Job drawing, mm, ordinate dimensions from the low corner. One solid piece. A direction names the side the tool comes from. Coordinates: 2 decimals unless noted, no trailing zeros. Write each loop counter-clockwise with the first axis right and the second up, starting at its lowest first coordinate (ties: lowest second). Pieces come first, ordered by that corner, then holes. Notation, with made-up numbers: (58.5, 74) - (77.5, 74) arc R17 ccw to (77.5, 93) - close; hole circle Ø3 at (52.25, -10). An arc over 180 degrees is marked (long way). Use one line per item in the form item = value. Start each with the question number.
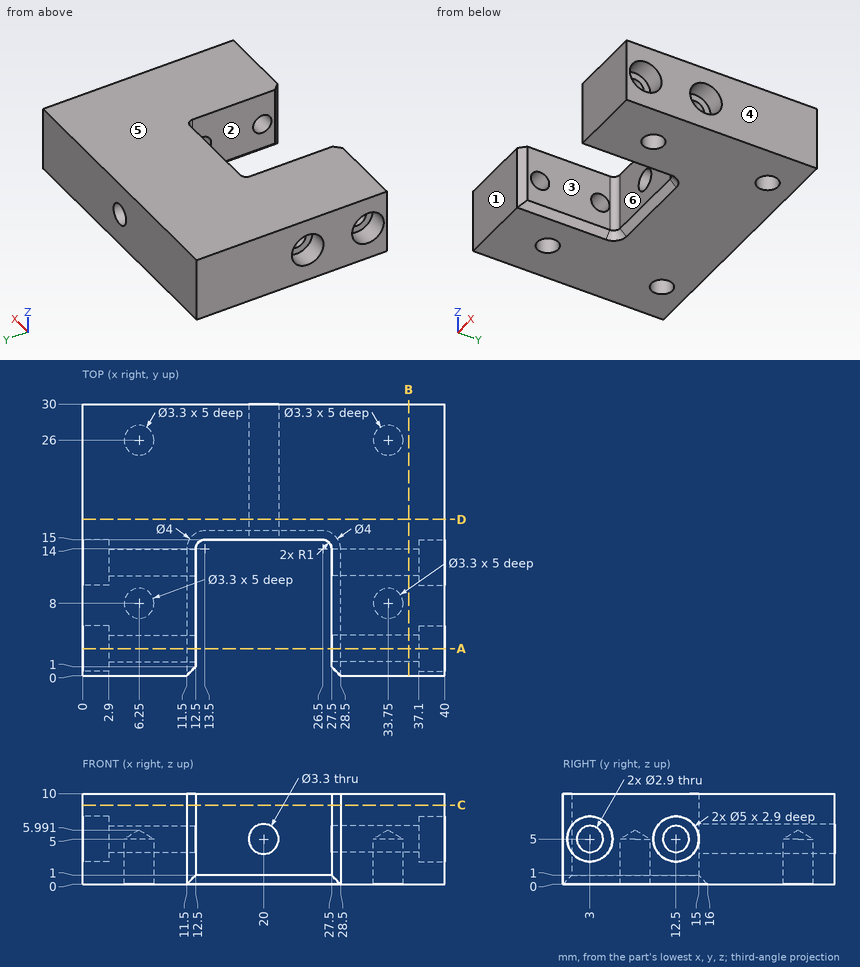
Q1. Which spindle directions (+Z, -Z, +X, -X, +Y, -Y) get a long thin tool onto all of the face, cutting with end or side? Do the marked faces 1 and 2. Say none if no direction does.
Q2. Pin check, flat tips, straight feed: P1, Ø4.5, axis at y = 12.5, z = 5, coming from the -X side; P2, Ø2.5, axis at y = 9.5, z = 6.5, coming from the -X side; P3, Ø2, axis at x = 6.25, y = 26, coming from the -Z side; P4, Ø5, axis at x = 21, z = 3.5, coming from the -Y side. Stop position of each tip, or through.
Q3. Slice it at B-B (x = 36). List the corners of the cut face in (y, z), plus the area to 3 significant figures.
Q4. Drill centre lines: probe 1 along Y at (x, z) = (29.5, 5); probe 2 along Y at (x, z) = (38.9, 5); probe 3 along X at (y, z) = (6.25, 5). Where is each one in solid material? Low to high.
Q5. Slice it at A-A (y = 3). List the corners of the cut face in (x, z), plus the area to 3 significant figures.
Q6. Slice it at D-D (y = 17.25). List the corners of the cut face in (x, z).
Q7. Slice it at C-C (z = 8.75). List the corners of the cut face in (x, y).
Q8. Mould opens along X. For the marked faces 3, 4, 5 and 6 say: released by +X, released by -X, zero draft, split by the parting line, or undercut.
Solution:
q1.face_1 = +Z, -Z, +X, -X, -Y
q1.face_2 = +Z, -Z, -Y
q2.P1 = 2.9
q2.P2 = 0
q2.P3 = 5.39
q2.P4 = 15
q3.outline = (0, 0) - (30, 0) - (30, 10) - (0, 10) - close; hole circle Ø2.9 at (3, 5); hole circle Ø2.9 at (12.5, 5)
q3.area = 287 mm2
q4.probe_1 = 0 to 1.55, 4.45 to 11.05, 13.95 to 30
q4.probe_2 = 0 to 0.5, 5.5 to 10, 15 to 30
q4.probe_3 = 0 to 12.5, 27.5 to 40
q5.outline = (0, 0) - (11.5, 0) - (12.5, 1) - (12.5, 3.55) - (2.9, 3.55) - (2.9, 2.5) - (0, 2.5) - close; (0, 7.5) - (2.9, 7.5) - (2.9, 6.45) - (12.5, 6.45) - (12.5, 10) - (0, 10) - close; (27.5, 1) - (28.5, 0) - (40, 0) - (40, 2.5) - (37.1, 2.5) - (37.1, 3.55) - (27.5, 3.55) - close; (27.5, 6.45) - (37.1, 6.45) - (37.1, 7.5) - (40, 7.5) - (40, 10) - (27.5, 10) - close
q5.area = 164 mm2
q6.outline = (0, 0) - (40, 0) - (40, 10) - (0, 10) - close; hole circle Ø3.3 at (20, 5)
q7.outline = (0, 0) - (11.5, 0) - (12.5, 1) - (12.5, 14) arc R1 cw to (13.5, 15) - (26.5, 15) arc R1 cw to (27.5, 14) - (27.5, 1) - (28.5, 0) - (40, 0) - (40, 30) - (0, 30) - close
q8.face_3 = undercut
q8.face_4 = released by +X
q8.face_5 = zero draft
q8.face_6 = undercut
